Model file for the job. Use its own axes, mm. Round coordinates to 2 decimals unless told otherwise and drop trailing zeros. Order: outer loops, then holes, each group sorted by start corner. A loop starts at its lowest first (then second) coordinate and runs counter-clockwise, first axis right, second up. Notation, with made-up numbers: (71, 0.25) -> (95, 0.25) arc R12 ccw to (95, 23.25) -> close; hole circle Ø4 at (33, -7.5). An arc over 180 degrees is marked (long way). Put each result on its own line as item: value. Start each with the question number.
Q1. Flat gauge pins, fed straight in: P1, Ø12, axis at x = 22.5, z = 7.5, coming from the -Y side; P2, Ø1, axis at y = -19.5, z = 3.5, coming from the +X side; P3, Ø2, axis at y = -49.5, z = -4.5, coming from the -X side. Where does each tip first touch, or does it go through?
Q2. Cut at A-A, the plane x = -4. List the corners of the cut face in (y, z).
Q3. Cut at B-B, the plane y = -80. List the corners of the cut face in (x, z), and give its area (3 significant figures).
Q4. Pull direction Z, two halves, no side cores. Call faces 1 (the face through (-2.601, -68.285, -20.916)), 2 (the face through (0, -80, -27)), 3 (the face through (-1, -65, 15)): released by +Z, released by -Z, zero draft, split by the parting line, or undercut.
Q5. Probe L1, parallel to Z at x = 2, y = -27.5; L2, parallel to Y at x = 3, z = -6.5; L3, parallel to X at y = -100, z = 6. List the from-to ranges inside material, lowest first.
Q6. Cut at D-D, the plane z = -19. List the corners of the cut face in (x, y).
Q7. Cut at C-C, the plane z = 1. List the corners of the cut face in (x, y).
from build123d import *

# Parameters (mm, degrees)
SALIENTE_EXTRUIR2_DEPTH = 15
CROQUIS2_R              = 12
SALIENTE_EXTRUIR3_DEPTH = 12


with BuildPart() as part:
    # Croquis1 → Saliente-Extruir2 (new, symmetric)
    with BuildSketch(Plane.XY):
        with BuildLine():
            Line((-17.305996071, 4.95), (-38.457769046, -69))
            ThreePointArc((-38.457769046, -69), (0, -120), (38.457769046, -69))
            Line((38.457769046, -69), (17.305996071, 4.95))
            ThreePointArc((17.305996071, 4.95), (0, 18), (-17.305996071, 4.95))
        make_face()
    extrude(amount=SALIENTE_EXTRUIR2_DEPTH, both=True)

    # Croquis2 → Saliente-Extruir3 (add)
    with BuildSketch(Plane(origin=(0, 0, -15), x_dir=(-1, 0, 0), z_dir=(0, 0, -1))):
        with Locations(Location((0, -80, 0), (0, 0, 180))):
            Circle(CROQUIS2_R)
    extrude(amount=SALIENTE_EXTRUIR3_DEPTH)


solid = part.part
Ans:
1. P1: stops at y = -116.44
1. P2: stops at x = 24.44
1. P3: stops at x = -33.17
2. outline: (-119.8, -15) -> (-91.31, -15) -> (-91.31, -27) -> (-68.69, -27) -> (-68.69, -15) -> (17.55, -15) -> (17.55, 15) -> (-119.8, 15) -> close
3. outline: (-40, -15) -> (-12, -15) -> (-12, -27) -> (12, -27) -> (12, -15) -> (40, -15) -> (40, 15) -> (-40, 15) -> close
3. area: 2,690 mm^2
4. face 1: zero draft
4. face 2: released by -Z
4. face 3: released by +Z
5. L1: z = -15 to 15
5. L2: y = -119.89 to 17.75
5. L3: x = -34.64 to 34.64
6. outline: circle Ø24 at (0, -80)
7. outline: (-38.46, -69) arc R40 ccw (long way) to (38.46, -69) -> (17.31, 4.95) arc R18 ccw to (-17.31, 4.95) -> close
